from build123d import *

# Parameters (mm, degrees)
F0_W     = 22.86
F0_H     = 22.86
F1_DEPTH = 3.81
F4_W     = 22.86
F4_H     = 22.86
F4_R     = 3.81
F5_DEPTH = 2.54


with BuildPart() as f1:
    # F0 (on Top) → F1 (new body)
    with BuildSketch(Plane.XY):
        Rectangle(F0_W, F0_H)
    extrude(amount=F1_DEPTH)

    # F2 (on Front) → F3 (revolve, cut)
    with BuildSketch(Plane.XZ):
        with BuildLine():
            Line((0, 3.81), (0, 0))
            Line((0, 0), (6.35, 0))
            ThreePointArc((6.35, 0), (9.044077, 1.115923), (10.16, 3.81))
            Line((10.16, 3.81), (0, 3.81))
        make_face()
    revolve(axis=Axis((0, 0, 1.905), (0, 0, 1)), mode=Mode.SUBTRACT)

    # F4 (on face) → F5 (join)
    with BuildSketch(Plane(origin=(0, 0, 0), x_dir=(1, 0, 0), z_dir=(0, 0, -1))):
        Rectangle(F4_W, F4_H)
        Circle(F4_R, mode=Mode.SUBTRACT)
    extrude(amount=F5_DEPTH)


solid = f1.part
The listing builds one solid part. Answer for the finished solid, in the listing's coordinates (mm). A direction names the side the tool comes from. Round coordinates to 2 decimals unless told otherwise and drop trailing zeros. Write each loop counter-clockwise with the first axis right and the second up, starting at its lowest first coordinate (ties: lowest second). Pieces come first, ordered by that corner, then holes. Notation, with made-up numbers: M 26.5,58 L 62.5,58 A31 ccw 62.5,82 Z; hole C -5.75,7 d6. An arc over 180 degrees is marked long. Write each question's results on one line, items separated by ' | '. Start each with the question number.
Item 1: A cutting plane is placed at C-C on z = -0.5. Write down the section's boundary in (x, y), and give its area (3 significant figures).
Item 2: Straight lines are drawn through the part: L1, parallel to X at y = 0, z = -1.2; L2, parallel to Z at x = 3, y = -4. For each, find the intervals that lie inside material, in ascending order. Write a range as [from, to].
Item 3: A cutting plane is placed at A-A on y = 0. Write down the section's boundary in (x, z), and give its area (3 significant figures).
Item 4: For faces 5 (the face through (3, 3, 0)), 6 (the face through (0, 11.43, 1)), determine the directions among +Z, -Z, +X, -X, +Y, -Y from which every point of the face is accessible in a straight line to the end or side of a thin tool.
Item 5: A flat-ended cylindrical pin translates along its axis: pin 1 Ø5 at (x, y) = (3, -3.5) entering from +Z. Find the tip coordinate at first contact, or state that the pin passes through.
Item 6: For a pull along X with two mould halves and no side action, classify faces 1 (the face through (-0.83, 3.72, -1.25)), 2 (the face through (11.43, 0, 1)), 3 (the face through (0, -11.43, 1)), 4 (the face through (-11.43, 0, 1)) as pulls with the +X half, pulls with the -X half, needs draft (parallel to the pull), parting line crosses it, or undercut.
Item 7: A cutting plane is placed at D-D on z = 1.5. Write down the section's boundary in (x, y).
Check sheet entries:
1) outline: M -11.43,-11.43 L 11.43,-11.43 L 11.43,11.43 L -11.43,11.43 Z; hole C 0,0 d7.62 | area: 477 mm²
2) L1: [-11.43, -3.81], [3.81, 11.43] | L2: [-2.54, 0]
3) outline: M -11.43,-2.54 L -3.81,-2.54 L -3.81,0 L -6.35,0 A3.81 cw -10.16,3.81 L -11.43,3.81 Z; M 3.81,-2.54 L 11.43,-2.54 L 11.43,3.81 L 10.16,3.81 A3.81 cw 6.35,0 L 3.81,0 Z | area: 54.6 mm²
4) face 5: +Z | face 6: +Z, -Z, +X, -X, +Y
5) pin 1: z = 0.08
6) face 1: undercut | face 2: pulls with the +X half | face 3: needs draft | face 4: pulls with the -X half
7) outline: M -11.43,-11.43 L 11.43,-11.43 L 11.43,11.43 L -11.43,11.43 Z; hole C 0,0 d18.76
